from build123d import *

# Parameters (mm, degrees)
SKETCH_1_R          = 16
EXTRUDE_1_DEPTH     = 5
SKETCH_2_R          = 16
EXTRUDE_2_DEPTH     = 2
SKETCH_3_R          = 1.6
CUT_EXTRUDE_1_DEPTH = 24.685438565


with BuildPart() as part:
    # 草图1 → 凸台-拉伸1 (new body)
    with BuildSketch(Plane(origin=(0, 0, 0), x_dir=(1, 0, 0), z_dir=(0, 1, 0))):
        with Locations(Location((0, 0, 0), (0, 0, 270))):
            Circle(SKETCH_1_R)
    extrude(amount=EXTRUDE_1_DEPTH)

    # 草图2 → 凸台-拉伸2 (add)
    with BuildSketch(Plane(origin=(0, 5, 0), x_dir=(1, 0, 0), z_dir=(0, 1, 0))):
        with Locations(Location((0, 0, 0), (0, 0, 270))):
            Circle(SKETCH_2_R)
    extrude(amount=EXTRUDE_2_DEPTH)

    # 草图3 → 切除-拉伸1 (cut, through all)
    with BuildSketch(Plane(origin=(0, 7, 0), x_dir=(1, 0, 0), z_dir=(0, 1, 0))):
        with Locations(Location((0, 12.5, 0), (0, 0, 270))):
            Circle(SKETCH_3_R)
        with Locations(Location((10.825317547, 6.25, 0), (0, 0, 270))):
            Circle(SKETCH_3_R)
        with Locations(Location((10.825317547, -6.25, 0), (0, 0, 270))):
            Circle(SKETCH_3_R)
        with Locations(Location((0, -12.5, 0), (0, 0, 270))):
            Circle(SKETCH_3_R)
        with Locations(Location((-10.825317547, -6.25, 0), (0, 0, 270))):
            Circle(SKETCH_3_R)
        with Locations(Location((-10.825317547, 6.25, 0), (0, 0, 270))):
            Circle(SKETCH_3_R)
    extrude(amount=-CUT_EXTRUDE_1_DEPTH, mode=Mode.SUBTRACT)


solid = part.part
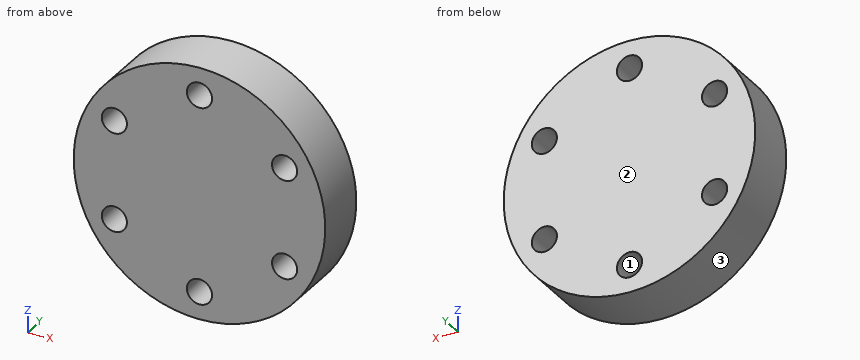
Could you check a few things on this model? Use its own coordinates, in mm. Face numbers are marked on the shaded views. Give positions to 0.01 mm unless a question says otherwise; leave off trailing zeros. Order: outer loops, then holes, each group sorted by start corner. A loop starts at its lowest first (then second) coordinate and runs counter-clockwise, first axis right, second up. Notation, with made-up numbers: (-36, 8.25) -> (-17, 8.25) arc R24 ccw to (-17, 37.25) -> close; hole circle Ø11 at (20, -22.5). An arc over 180 degrees is marked (long way). Answer in a Markdown table with one row per item. Add a question column.
Item 1: Imagine slicing it at C-C (y = 0.75). List the corners of the cut face in (x, z) for me.
Item 2: Imagine slicing it at B-B (z = 6.25). List the corners of the cut face in (x, y) for me.
Item 3: Imagine slicing it at A-A (x = 0). List the corners of the cut face in (y, z) for me, and give its area (3 significant figures).
Item 4: I'm going to push a flat-ended pin straight in: P1, Ø3, axis at x = 5, y = 2, coming from the +Z side. Where does the tip first touch, or does it pass through?
Item 5: Please list where these lines run through material, in increasing order: probe 1 along X at (y, z) = (4.5, 6.25); probe 2 along Z at (x, y) = (-10, 3.25); probe 3 along Z at (x, y) = (10.5, 5.25).
Item 6: Imagine slicing it at D-D (z = 12.5). List the corners of the cut face in (x, y) for me.
Item 7: We'd pull the mould along Z, two halves only. Please class the marked faces 1, 2 and 3: pulls with the +Z half, pulls with the -Z half, needs draft (parallel to the pull), parting line crosses it, or undercut.
Result:
| question | item | result |
|---|---|---|
| 1 | outline | circle Ø32 at (0, 0); hole circle Ø3.2 at (-10.83, -6.25); hole circle Ø3.2 at (-10.83, 6.25); hole circle Ø3.2 at (0, -12.5); hole circle Ø3.2 at (0, 12.5); hole circle Ø3.2 at (10.83, -6.25); hole circle Ø3.2 at (10.83, 6.25) |
| 2 | outline | (-14.73, 0) -> (-12.43, 0) -> (-12.43, 7) -> (-14.73, 7) -> close; (-9.23, 0) -> (9.23, 0) -> (9.23, 7) -> (-9.23, 7) -> close; (12.43, 0) -> (14.73, 0) -> (14.73, 7) -> (12.43, 7) -> close |
| 3 | outline | (0, -16) -> (7, -16) -> (7, -14.1) -> (0, -14.1) -> close; (0, -10.9) -> (7, -10.9) -> (7, 10.9) -> (0, 10.9) -> close; (0, 14.1) -> (7, 14.1) -> (7, 16) -> (0, 16) -> close |
| 3 | area | 179 mm2 |
| 4 | P1 | z = 15.61 |
| 5 | probe 1 | -14.73 to -12.43, -9.23 to 9.23, 12.43 to 14.73 |
| 5 | probe 2 | -12.49 to -7.62, -4.88 to 4.88, 7.62 to 12.49 |
| 5 | probe 3 | -12.07 to -7.82, -4.68 to 4.68, 7.82 to 12.07 |
| 6 | outline | (-9.99, 0) -> (-1.6, 0) -> (-1.6, 7) -> (-9.99, 7) -> close; (1.6, 0) -> (9.99, 0) -> (9.99, 7) -> (1.6, 7) -> close |
| 7 | face 1 | undercut |
| 7 | face 2 | needs draft |
| 7 | face 3 | parting line crosses it |
